Check sheet for the modelled part. Datum: model origin and axes. Units: mm. A direction names the side the tool comes from. Give positions to 0.01 mm unless a question says otherwise; leave off trailing zeros. Loops run counter-clockwise (first coordinate to the right, second up) from the corner with the lowest first, then second, coordinate; pieces in that order, holes last. Notation, with made-up numbers: M -14,36 L 41,36 A8 ccw 41,46 Z; hole C 45,74 d10. An arc over 180 degrees is marked long. Put each result on its own line as item: value. Start each with the question number.
```python
from build123d import *

# Parameters (mm, degrees)
F1_DEPTH = 8
F2_DEPTH = 6
F3_DEPTH = 13
F6_DEPTH = 8
F6_TAPER = 15
F7_DEPTH = 3
F8_R     = 5
F9_R     = 1.99999


# Not quite as in the source:
# - a fillet or chamfer is up to 0.001 mm smaller than in the source, because OpenCascade refuses the exact size


with BuildPart() as f1:
    # F0 (on Front) → F1 (new body)
    with BuildSketch(Plane.XZ):
        Polygon((-13.4350288425, 13.4350288425), (0, 0), (13.4350288425, 13.4350288425), (3.7486736477, 13.4350288425), (2.0784609691, 10.5421356237), (-2.0784609691, 10.5421356237), (-3.7486736477, 13.4350288425), align=None)
        Polygon((3.7486736477, 13.4350288425), (13.4350288425, 13.4350288425), (0, 26.8700576851), (-13.4350288425, 13.4350288425), (-3.7486736477, 13.4350288425), (-4.1569219382, 14.1421356237), (-2.0784609691, 17.7421356237), (2.0784609691, 17.7421356237), (4.1569219382, 14.1421356237), align=None)
        Polygon((-11.313708499, 0), (0, 0), (-13.4350288425, 13.4350288425), (-19.091883092, 7.7781745931), align=None)
        Polygon((13.4350288425, 13.4350288425), (0, 0), (11.313708499, 0), (19.091883092, 7.7781745931), align=None)
        with BuildLine():
            Line((1.8708286934, 13.4350288425), (3.7486736477, 13.4350288425))
            Line((3.7486736477, 13.4350288425), (4.1569219382, 14.1421356237))
            Line((4.1569219382, 14.1421356237), (2.0784609691, 17.7421356237))
            Line((2.0784609691, 17.7421356237), (-2.0784609691, 17.7421356237))
            Line((-2.0784609691, 17.7421356237), (-4.1569219382, 14.1421356237))
            Line((-4.1569219382, 14.1421356237), (-3.7486736477, 13.4350288425))
            Line((-3.7486736477, 13.4350288425), (-1.8708286934, 13.4350288425))
            ThreePointArc((-1.8708286934, 13.4350288425), (-0.3594040993, 16.109577794), (2, 14.1421356237))
            ThreePointArc((2, 14.1421356237), (1.9674421703, 13.7827315244), (1.8708286934, 13.4350288425))
        make_face()
        with BuildLine():
            Line((2.0784609691, 10.5421356237), (3.7486736477, 13.4350288425))
            Line((3.7486736477, 13.4350288425), (1.8708286934, 13.4350288425))
            ThreePointArc((1.8708286934, 13.4350288425), (0, 12.1421356237), (-1.8708286934, 13.4350288425))
            Line((-1.8708286934, 13.4350288425), (-3.7486736477, 13.4350288425))
            Line((-3.7486736477, 13.4350288425), (-2.0784609691, 10.5421356237))
            Line((-2.0784609691, 10.5421356237), (2.0784609691, 10.5421356237))
        make_face()
    extrude(amount=-F1_DEPTH)

    # F0 (on Front) → F2 (cut)
    with BuildSketch(Plane.XZ):
        with BuildLine():
            Line((1.8708286934, 13.4350288425), (3.7486736477, 13.4350288425))
            Line((3.7486736477, 13.4350288425), (4.1569219382, 14.1421356237))
            Line((4.1569219382, 14.1421356237), (2.0784609691, 17.7421356237))
            Line((2.0784609691, 17.7421356237), (-2.0784609691, 17.7421356237))
            Line((-2.0784609691, 17.7421356237), (-4.1569219382, 14.1421356237))
            Line((-4.1569219382, 14.1421356237), (-3.7486736477, 13.4350288425))
            Line((-3.7486736477, 13.4350288425), (-1.8708286934, 13.4350288425))
            ThreePointArc((-1.8708286934, 13.4350288425), (-0.3594040993, 16.109577794), (2, 14.1421356237))
            ThreePointArc((2, 14.1421356237), (1.9674421703, 13.7827315244), (1.8708286934, 13.4350288425))
        make_face()
        with BuildLine():
            Line((2.0784609691, 10.5421356237), (3.7486736477, 13.4350288425))
            Line((3.7486736477, 13.4350288425), (1.8708286934, 13.4350288425))
            ThreePointArc((1.8708286934, 13.4350288425), (0, 12.1421356237), (-1.8708286934, 13.4350288425))
            Line((-1.8708286934, 13.4350288425), (-3.7486736477, 13.4350288425))
            Line((-3.7486736477, 13.4350288425), (-2.0784609691, 10.5421356237))
            Line((-2.0784609691, 10.5421356237), (2.0784609691, 10.5421356237))
        make_face()
    extrude(amount=-F2_DEPTH, mode=Mode.SUBTRACT)

    # F0 (on Front) → F3 (join)
    with BuildSketch(Plane.XZ):
        Polygon((-11.313708499, 0), (0, 0), (-13.4350288425, 13.4350288425), (-19.091883092, 7.7781745931), align=None)
        Polygon((-13.4350288425, 13.4350288425), (0, 0), (13.4350288425, 13.4350288425), (3.7486736477, 13.4350288425), (2.0784609691, 10.5421356237), (-2.0784609691, 10.5421356237), (-3.7486736477, 13.4350288425), align=None)
        Polygon((13.4350288425, 13.4350288425), (0, 0), (11.313708499, 0), (19.091883092, 7.7781745931), align=None)
        with BuildLine():
            ThreePointArc((-1.8708286934, 13.4350288425), (0, 12.1421356237), (1.8708286934, 13.4350288425))
            Line((1.8708286934, 13.4350288425), (0, 13.4350288425))
            Line((0, 13.4350288425), (-1.8708286934, 13.4350288425))
        make_face()
        with BuildLine():
            Line((2.0784609691, 10.5421356237), (3.7486736477, 13.4350288425))
            Line((3.7486736477, 13.4350288425), (1.8708286934, 13.4350288425))
            ThreePointArc((1.8708286934, 13.4350288425), (0, 12.1421356237), (-1.8708286934, 13.4350288425))
            Line((-1.8708286934, 13.4350288425), (-3.7486736477, 13.4350288425))
            Line((-3.7486736477, 13.4350288425), (-2.0784609691, 10.5421356237))
            Line((-2.0784609691, 10.5421356237), (2.0784609691, 10.5421356237))
        make_face()
    extrude(amount=F3_DEPTH)

    # F5 (on offset) → F6 (cut)
    with BuildSketch(Plane.XZ.offset(8)):
        with BuildLine():
            Line((0, 26.8700576851), (-13.4350288425, 13.4350288425))
            Line((-13.4350288425, 13.4350288425), (-3.5355339059, 3.5355339059))
            ThreePointArc((-3.5355339059, 3.5355339059), (0, 2.0710678119), (3.5355339059, 3.5355339059))
            Line((3.5355339059, 3.5355339059), (13.4350288425, 13.4350288425))
            Line((13.4350288425, 13.4350288425), (0, 26.8700576851))
        make_face()
    extrude(amount=-F6_DEPTH, taper=F6_TAPER, mode=Mode.SUBTRACT)

    # F5 (on offset) → F7 (cut)
    with BuildSketch(Plane.XZ.offset(8)):
        with BuildLine():
            Line((0, 26.8700576851), (-13.4350288425, 13.4350288425))
            Line((-13.4350288425, 13.4350288425), (-3.5355339059, 3.5355339059))
            ThreePointArc((-3.5355339059, 3.5355339059), (0, 2.0710678119), (3.5355339059, 3.5355339059))
            Line((3.5355339059, 3.5355339059), (13.4350288425, 13.4350288425))
            Line((13.4350288425, 13.4350288425), (0, 26.8700576851))
        make_face()
    extrude(amount=F7_DEPTH, mode=Mode.SUBTRACT)

    # F8
    f8_edges = [f1.edges().sort_by_distance(p)[0] for p in [
        (-19.091883, -2.5, 7.778175),
        (0, 4, 26.870058),
        (19.091883, -2.5, 7.778175),
    ]]
    fillet(f8_edges, radius=F8_R)

    # F9 (radius 2 in the source; OpenCascade refuses exactly that, so slightly less here)
    f9_edges = [f1.edges().sort_by_distance(p)[0] for p in [
        (-14.495689, -13, 12.374369),
        (-17.020815, -13, 7.778175),
        (0, -13, 13.435029),
        (-13.435029, -13, 2.12132),
        (14.495689, -13, 12.374369),
        (0, -13, 0),
        (17.020815, -13, 7.778175),
        (13.435029, -13, 2.12132),
    ]]
    fillet(f9_edges, radius=F9_R)


solid = f1.part
```
Q1. Thickness scan on line 1 along Z through (x, y) = (0, 6.45); line 2 along Y through (x, z) = (6, 14.75); line 3 along Z through (x, y) = (-2.5, 5.5). Record the ranges inside material, lowest first. Write a range as [from, to].
Q2. Mould release check, pull along X, two halves, no side actions. Record for faces 1 (the face through (0, 8, 10)), 2 (the face through (-17.02, -1.37, 7.72)), 3 (the face through (-3.1, 2.96, 15.97)): pulls with the +X half, pulls with the -X half, needs draft (parallel to the pull), parting line crosses it, or undercut.
Q3. Section check C-C, the plane y = 4.75. Record the cut outline in (x, z).
Q4. Section check D-D, the plane y = -9. Record the cut outline in (x, z), then the cut area to 3 significant figures.
Q5. Depth check by flat-ended pin: P1, Ø1.5, axis at x = -11.5, y = -3, coming from the +Z side (3 decimals); P2, Ø4, axis at y = 0.5, z = 14, coming from the +X side; P3, Ø2, axis at x = 0, z = 13, coming from the -Y side. Enter the tip coordinate at first touch or a pass-through.
Q6. Section check B-B, the plane z = 14.75. Record the cut outline in (x, y), then the cut area to 3 significant figures.
Q7. Access from +Z, -Z, +X, -X, +Y, -Y to the whole of each face (thin tool, end or side, straight path). Record for faces 4 (the face through (0, 3, 17.742)), 5 (the face through (0, 3, 10.542)), 6 (the face through (-0.05, -9.48, 2.07)).
Found:
1. line 1: z = [0, 12.14], [16.14, 24.8]
1. line 2: y = [0, 8]
1. line 3: z = [0, 11.27], [17.01, 24.13]
2. face 1: needs draft
2. face 2: pulls with the -X half
2. face 3: undercut
3. outline: M -15.56,4.24 L -11.31,0 L 11.31,0 L 15.56,4.24 A5 ccw 15.56,11.31 L 3.54,23.33 A5 ccw -3.54,23.33 L -15.56,11.31 A5 ccw Z; hole M -4.16,14.14 L -2.08,10.54 L 2.08,10.54 L 4.16,14.14 L 2.08,17.74 L -2.08,17.74 Z
4. outline: M -15.56,4.24 L -11.31,0 L 11.31,0 L 15.56,4.24 A5 ccw 15.56,11.31 L 13.44,13.44 L 3.54,3.54 A5 cw -3.54,3.54 L -13.44,13.44 L -15.56,11.31 A5 ccw Z
4. area: 235 mm^2
5. P1: stops at z = 13.435
5. P2: stops at x = 14.87
5. P3: stops at y = -12.92
6. outline: M -12.12,0 L -3.81,0 L -3.81,6 L -1.91,6 L -1.91,8 L -12.12,8 Z; M 1.91,6 L 3.81,6 L 3.81,0 L 12.12,0 L 12.12,8 L 1.91,8 Z
6. area: 141 mm^2
7. face 4: -Y
7. face 5: none
7. face 6: +Z
